CAD build for the part. Positions are in the model's coordinates, mm. A direction names the side the tool comes from. Give positions to 0.01 mm unless a question says otherwise; leave off trailing zeros. Write each loop counter-clockwise with the first axis right and the second up, starting at its lowest first coordinate (ties: lowest second). Pieces come first, ordered by that corner, then holes. Notation, with made-up numbers: (78.5, 67.5) -> (82.5, 67.5) arc R18 ccw to (82.5, 84.5) -> close; hole circle Ø11 at (-28.5, 78). An arc over 180 degrees is marked (long way). Use one line per item in the form item = value. Start each with the question number.
from build123d import *

# Parameters (mm, degrees)
ESQUISSE1_W             = 190
ESQUISSE1_H             = 220
BOSS_EXTRU_1_DEPTH      = 31
ESQUISSE2_R             = 65
ENL_V_MAT_EXTRU_1_DEPTH = 38
ESQUISSE3_R             = 5
ENL_V_MAT_EXTRU_2_DEPTH = 30
ESQUISSE4_W             = 150
ESQUISSE4_H             = 150
ESQUISSE4_R             = 55
BOSS_EXTRU_2_DEPTH      = 10
CONG_1_R                = 2
CONG_2_R                = 2


with BuildPart() as part:
    # Esquisse1 → Boss.-Extru.1 (new body)
    with BuildSketch(Plane.XY):
        with Locations((0, 110)):
            Rectangle(ESQUISSE1_W, ESQUISSE1_H)
    extrude(amount=-BOSS_EXTRU_1_DEPTH)

    # Esquisse2 → Enlèv. mat.-Extru.1 (cut)
    with BuildSketch(Plane.XY):
        with Locations((0, 95)):
            Circle(ESQUISSE2_R)
    extrude(amount=-ENL_V_MAT_EXTRU_1_DEPTH, mode=Mode.SUBTRACT)

    # Esquisse3 → Enlèv. mat.-Extru.2 (cut)
    with BuildSketch(Plane(origin=(0, 220, 0), x_dir=(1, 0, 0), z_dir=(0, 1, 0))):
        with Locations(Location((-80, 15.5, 0), (0, 0, 270))):
            Circle(ESQUISSE3_R)
    enl_v_mat_extru_2 = extrude(amount=-ENL_V_MAT_EXTRU_2_DEPTH, mode=Mode.SUBTRACT)

    # Symétrie1: Enlèv. mat.-Extru.2 across plane
    add(enl_v_mat_extru_2.mirror(Plane(origin=(0, 0, 0), x_dir=(0, 0, 1), z_dir=(1, 0, 0))), mode=Mode.SUBTRACT)

    # Esquisse4 → Boss.-Extru.2 (add)
    with BuildSketch(Plane(origin=(0, 0, -31), x_dir=(-1, 0, 0), z_dir=(0, 0, -1))):
        with Locations((0, 95)):
            Rectangle(ESQUISSE4_W, ESQUISSE4_H)
        with Locations((0, 95)):
            Circle(ESQUISSE4_R, mode=Mode.SUBTRACT)
    extrude(amount=BOSS_EXTRU_2_DEPTH)

    # Congé1
    cong_1_edges = [part.edges().sort_by_distance(p)[0] for p in [
        (-75, 95, -31),
        (0, 170, -31),
        (75, 95, -31),
        (0, 20, -31),
    ]]
    fillet(cong_1_edges, radius=CONG_1_R)

    # Congé2
    cong_2_edges = [part.edges().sort_by_distance(p)[0] for p in [
        (55, 95, -41),
    ]]
    fillet(cong_2_edges, radius=CONG_2_R)


solid = part.part
1) Two-plate mould, pull along X, no slides. Class faces 1 (the face through (-84.88, 205.21, -16.58)), 2 (the face through (-14.091, 31.546, -15.283)), 3 (the face through (-32, 146, -41)), 4 (the face through (75, 94, -37)): released by +X, released by -X, zero draft, split by the parting line, or undercut.
2) Cut at B-B (x = -69). Give the cut face in (y, z).
3) Pin check, flat tips, straight feed: pin 1 (9 mm diameter, centred on x = -80, z = -15.5, fed in from +Y); pin 2 (4 mm diameter, centred on y = 89, z = -35.5, fed in from +X); pin 3 (9 mm diameter, centred on x = -4.5, z = -37.5, fed in from +Y). Stop position of each tip, or through.
4) 3-axis set-ups, long thin cutter, end or side, ignore diameter. For faces 5 (the face through (80, 190, -16)), 6 (the face through (-75, 94, -37)), 7 (the face through (1, 170, -37)): which of +Z, -Z, +X, -X, +Y, -Y reach the whole face in a straight line?
5) Cut at C-C (x = 0). Give the cut face in (y, z).
6) Wall check: line 1 along X through (y, z) = (210, -15); line 2 along Y through (x, z) = (0, -33.75); line 3 along Y through (x, z) = (0, -21). Give the ranges that are in metal, low to high. Write a range as from..to.
7) Cut at D-D (z = -26). Give the cut face in (x, y).
8) Cut at A-A (y = 95). Give the cut face in (x, z), and give its area (3 significant figures).
Final values:
q1.face_1 = undercut
q1.face_2 = undercut
q1.face_3 = zero draft
q1.face_4 = released by +X
q2.outline = (0, -31) -> (18, -31) arc R2 cw to (20, -33) -> (20, -41) -> (170, -41) -> (170, -33) arc R2 cw to (172, -31) -> (220, -31) -> (220, 0) -> (0, 0) -> close
q3.pin_1 = 190
q3.pin_2 = 75
q3.pin_3 = 170
q4.face_5 = +Y
q4.face_6 = -Z, -X, +Y, -Y
q4.face_7 = -Z, +X, -X, +Y
q5.outline = (0, -31) -> (18, -31) arc R2 cw to (20, -33) -> (20, -41) -> (38, -41) arc R2 ccw to (40, -39) -> (40, -31) -> (30, -31) -> (30, 0) -> (0, 0) -> close; (150, -39) arc R2 ccw to (152, -41) -> (170, -41) -> (170, -33) arc R2 cw to (172, -31) -> (220, -31) -> (220, 0) -> (160, 0) -> (160, -31) -> (150, -31) -> close
q6.line_1 = -95..-84.97, -75.03..75.03, 84.97..95
q6.line_2 = 20..40, 150..170
q6.line_3 = 0..30, 160..220
q7.outline = (-95, 0) -> (95, 0) -> (95, 220) -> (-95, 220) -> close; hole circle Ø130 at (0, 95)
q8.outline = (-95, -31) -> (-77, -31) arc R2 cw to (-75, -33) -> (-75, -41) -> (-57, -41) arc R2 ccw to (-55, -39) -> (-55, -31) -> (-65, -31) -> (-65, 0) -> (-95, 0) -> close; (55, -39) arc R2 ccw to (57, -41) -> (75, -41) -> (75, -33) arc R2 cw to (77, -31) -> (95, -31) -> (95, 0) -> (65, 0) -> (65, -31) -> (55, -31) -> close
q8.area = 2,260 mm^2
